from build123d import *

# Parameters (mm, degrees)
SKIZZE2_W               = 6
SKIZZE2_H               = 6
LINEAR_AUSTRAGEN1_DEPTH = 4.6
SKIZZE3_R               = 3
LINEAR_AUSTRAGEN2_DEPTH = 15.4
FASE1_SIZE              = 0.5


with BuildPart() as part:
    # Skizze1 → Rotation1 (revolve)
    with BuildSketch(Plane(origin=(0, 0, 0), x_dir=(1, 0, 0), z_dir=(0, 1, 0))):
        with BuildLine():
            Line((0, 0), (0, 8.275))
            ThreePointArc((0, 8.275), (-2.861847997, 4.569738094), (-3.88, 0))
            Line((-3.88, 0), (0, 0))
        make_face()
    revolve(axis=Axis((0, 0, 0), (-1, 0, 0)))

    # Skizze2 → Linear austragen1 (add)
    with BuildSketch(Plane(origin=(0, 0, 0), x_dir=(0, 0, -1), z_dir=(1, 0, 0))):
        Rectangle(SKIZZE2_W, SKIZZE2_H)
    extrude(amount=LINEAR_AUSTRAGEN1_DEPTH)

    # Skizze3 → Linear austragen2 (add)
    with BuildSketch(Plane(origin=(4.6, 0, 0), x_dir=(0, 0, -1), z_dir=(1, 0, 0))):
        Circle(SKIZZE3_R)
    extrude(amount=LINEAR_AUSTRAGEN2_DEPTH)

    # Fase1
    fase1_edges = [part.edges().sort_by_distance(p)[0] for p in [
        (20, 0, 3),
    ]]
    chamfer(fase1_edges, length=FASE1_SIZE)


solid = part.part
Work out the finished part from the listing and answer in its coordinate system (mm). A direction names the side the tool comes from. Round coordinates to 2 decimals unless told otherwise and drop trailing zeros. Write each loop counter-clockwise with the first axis right and the second up, starting at its lowest first coordinate (ties: lowest second). Pieces come first, ordered by that corner, then holes. Notation, with made-up numbers: (0, 47.25) - (34, 47.25) arc R33 cw to (34, 84.25) - close; hole circle Ø3 at (-3, 8). An arc over 180 degrees is marked (long way). Answer in a Markdown table with one row per item. Add a question column.
1. Find the intervals of material crossed by line 1 along Y through (x, z) = (15.25, 0); line 2 along X through (y, z) = (-4.75, -6.25); line 3 along X through (y, z) = (-0.5, -2.25), in increasing order. Write a range as from..to.
2. The mould has two halves that part along Z. Classify faces 5 (the flat face through (2, 0, -3)), 6 (the flat face through (2, 0, 3)), 7 (the flat face through (0, 0, 4)): +Z half, -Z half, draft (parallel to the pull), parting line (faces both ways), or undercut.
3. A cutting plane is placed at C-C, the plane z = 6.5. Determine the outline of the cut face in (x, y), and give its area (3 significant figures).
4. A cutting plane is placed at B-B, the plane y = -5. Determine the outline of the cut face in (x, z).
5. Given pin 1 (2.5 mm diameter, centred on x = 2, z = 1.5, fed in from -Y); pin 2 (4 mm diameter, centred on x = 15, z = -3, fed in from -Y); pin 3 (1.4 mm diameter, centred on x = 1.5, y = -0.5, fed in from +Z), each flat-ended and moving along its own axis, determine where each tip first touches the part or whether it passes through.
6. A cutting plane is placed at A-A, the plane x = 1.75. Determine the outline of the cut face in (y, z), and give its area (3 significant figures).
7. For faces 1 (the flat face through (4.6, 2.4, -2.3)), 2 (the cylindrical face through (12, 0, 3)), 3 (the flat face through (2, 3, 0)), 4 (the flat face through (2, -3, 0)), determine the directions among +Z, -Z, +X, -X, +Y, -Y from which every point of the face is accessible in a straight line to the end or side of a thin tool.
8. A cutting plane is placed at D-D, the plane x = 17.5. Determine the outline of the cut face in (y, z).
Worked out:
| question | item | result |
|---|---|---|
| 1 | line 1 | -3..3 |
| 1 | line 2 | -0.48..0 |
| 1 | line 3 | -3.63..20 |
| 2 | face 5 | -Z half |
| 2 | face 6 | +Z half |
| 2 | face 7 | draft |
| 3 | outline | (0, -5.12) - (0, 5.12) arc R8.58 ccw to start |
| 3 | area | 11.8 mm^2 |
| 4 | outline | (0, -6.59) - (0, 6.59) arc R9.53 ccw to start |
| 5 | pin 1 | y = -3 |
| 5 | pin 2 | y = -2.83 |
| 5 | pin 3 | z = 3 |
| 6 | outline | (-3, -3) - (3, -3) - (3, 3) - (-3, 3) - close |
| 6 | area | 36.0 mm^2 |
| 7 | face 1 | -Z, +X, +Y |
| 7 | face 2 | +X |
| 7 | face 3 | +Z, -Z, +X, +Y |
| 7 | face 4 | +Z, -Z, +X, -Y |
| 8 | outline | circle Ø6 at (0, 0) |
